from build123d import *

# Parameters (mm, degrees)
SKETCH1_W              = 19.05
SKETCH1_H              = 19.05
BOSS_EXTRUDE1_DEPTH    = 50.8
CUT_EXTRUDE1_DEPTH     = 12.7
F_8_CLEARANCE_HOLE1_D  = 4.4958
FILLET1_R              = 0.381
F_10_32_TAPPED_HOLE1_D = 4.0386
FILLET2_R              = 5.08


with BuildPart() as part:
    # Sketch1 → Boss-Extrude1 (new body)
    with BuildSketch(Plane.XY):
        Rectangle(SKETCH1_W, SKETCH1_H)
    extrude(amount=BOSS_EXTRUDE1_DEPTH)

    # Sketch2 → Cut-Extrude1 (cut)
    with BuildSketch(Plane.XZ.offset(9.525)):
        with BuildLine():
            Line((-0.79375, 47.625), (0.79375, 47.625))
            ThreePointArc((0.79375, 47.625), (3.03881403, 46.69506403), (3.96875, 44.45))
            Line((3.96875, 44.45), (3.96875, 38.1))
            ThreePointArc((3.96875, 38.1), (3.03881403, 35.85493597), (0.79375, 34.925))
            Line((0.79375, 34.925), (-0.79375, 34.925))
            ThreePointArc((-0.79375, 34.925), (-3.03881403, 35.85493597), (-3.96875, 38.1))
            Line((-3.96875, 38.1), (-3.96875, 44.45))
            ThreePointArc((-3.96875, 44.45), (-3.03881403, 46.69506403), (-0.79375, 47.625))
        make_face()
    extrude(amount=-CUT_EXTRUDE1_DEPTH, mode=Mode.SUBTRACT)

    # #8 Clearance Hole1 (through all)
    with Locations(Plane(origin=(0, 3.175, 0), x_dir=(-1, 0, 0), z_dir=(0, -1, 0))):
        with Locations((0, -41.275)):
            Hole(F_8_CLEARANCE_HOLE1_D / 2)

    # Fillet1
    fillet1_edges = [part.edges().sort_by_distance(p)[0] for p in [
        (0, -9.525, 47.625),
        (3.96875, -9.525, 41.275),
        (-3.03881403, -9.525, 46.69506403),
        (-3.96875, -9.525, 41.275),
        (-3.03881403, -9.525, 35.85493597),
        (0, -9.525, 34.925),
        (3.03881403, -9.525, 35.85493597),
        (3.03881403, -9.525, 46.69506403),
    ]]
    fillet(fillet1_edges, radius=FILLET1_R)

    # #10-32 Tapped Hole1 (through all)
    with Locations(Plane(origin=(0, 9.525, 0), x_dir=(1, 0, 0), z_dir=(0, 1, 0))):
        with Locations((0, -12.7)):
            Hole(F_10_32_TAPPED_HOLE1_D / 2)

    # Fillet2
    fillet2_edges = [part.edges().sort_by_distance(p)[0] for p in [
        (9.525, -9.525, 25.4),
        (-9.525, -9.525, 25.4),
        (-9.525, 9.525, 25.4),
        (9.525, 9.525, 25.4),
    ]]
    fillet(fillet2_edges, radius=FILLET2_R)


solid = part.part
Design review of the part built by this model. Coordinates are the model's own, in mm. A direction names the side the tool comes from. Give positions to 0.01 mm unless a question says otherwise; leave off trailing zeros. Loops run counter-clockwise (first coordinate to the right, second up) from the corner with the lowest first, then second, coordinate; pieces in that order, holes last. Notation, with made-up numbers: (12.25, 9) -> (45.25, 9) arc R11 cw to (45.25, 22) -> close; hole circle Ø2 at (0.25, 50.25). An arc over 180 degrees is marked (long way). One line per question, with ' | ' between items. Start each with the question number.
(1) For faces 1 (the face through (-3.063, -3.071, 46.67)), 2 (the face through (0, 0, 50.8)), list the 3-axis set-ups (+Z, -Z, +X, -X, +Y, -Y) from which the entire face can be reached by the end or side of a thin tool; tool diameter is ignored.
(2) Draft analysis for pull direction Z (two halves, no side actions). For faces 3 (the face through (-9.525, 0, 25)), 4 (the face through (0, 0, 0)), 5 (the face through (-2, 3.175, 43)), state which applies: +Z half, -Z half, draft (parallel to the pull), parting line (faces both ways), or undercut.
(3) We need section C-C (y = 7.75). State the section outline as (x, z) points (3 decimals).
(4) Insertion check: P1, Ø7, axis at x = 0, z = 41.275, coming from the -Y side (3 decimals); P2, Ø3, axis at y = -7.5, z = 35, coming from the +X side. Each pin has a flat end and moves straight along its axis. Give the tip position at first contact, or say it passes through.
(5) We need section D-D (x = 6). State the section outline as (y, z) points, and give its area (3 significant figures).
(6) We need section B-B (x = 0). State the section outline as (y, z) points (3 decimals), and give its area (3 significant figures).
(7) For line 1 (Z direction, x = 0, y = 5); line 2 (X direction, y = 1.25, z = 12.7) (3 decimals); line 3 (Z direction, x = 0.5, y = -8.5) (3 decimals), list the stretches that pass through material, from the lowest coordinate up.
(8) We need section A-A (z = 12.7). State the section outline as (x, y) points (3 decimals), and give its area (3 significant figures).
The answers:
1) face 1: -Y | face 2: +Z, +X, -X, +Y, -Y
2) face 3: draft | face 4: -Z half | face 5: undercut
3) outline: (-8.303, 0) -> (8.303, 0) -> (8.303, 50.8) -> (-8.303, 50.8) -> close; hole circle Ø4.496 at (0, 41.275); hole circle Ø4.039 at (0, 12.7)
4) P1: stops at y = 3.175 | P2: stops at x = 9.28
5) outline: (-9.28, 0) -> (9.28, 0) -> (9.28, 50.8) -> (-9.28, 50.8) -> close | area: 943 mm^2
6) outline: (-9.525, 0) -> (9.525, 0) -> (9.525, 10.681) -> (-9.525, 10.681) -> close; (-9.525, 14.719) -> (9.525, 14.719) -> (9.525, 39.027) -> (3.175, 39.027) -> (3.175, 34.925) -> (-9.144, 34.925) arc R0.381 ccw to (-9.525, 34.544) -> close; (-9.525, 48.006) arc R0.381 ccw to (-9.144, 47.625) -> (3.175, 47.625) -> (3.175, 43.523) -> (9.525, 43.523) -> (9.525, 50.8) -> (-9.525, 50.8) -> close | area: 701 mm^2
7) line 1: z = 0 to 10.68, 14.72 to 39.03, 43.52 to 50.8 | line 2: x = -9.525 to -2.019, 2.019 to 9.525 | line 3: z = 0 to 10.744, 14.656 to 34.925, 47.625 to 50.8
8) outline: (-9.525, -4.445) arc R5.08 ccw to (-4.445, -9.525) -> (-2.019, -9.525) -> (-2.019, 9.525) -> (-4.445, 9.525) arc R5.08 ccw to (-9.525, 4.445) -> close; (2.019, -9.525) -> (4.445, -9.525) arc R5.08 ccw to (9.525, -4.445) -> (9.525, 4.445) arc R5.08 ccw to (4.445, 9.525) -> (2.019, 9.525) -> close | area: 264 mm^2
